Source: CAD feature listing. Evaluate the final solid. Frame: model axes, mm. A direction names the side the tool comes from. Coordinates: 2 decimals unless noted, no trailing zeros. Loops run counter-clockwise (first coordinate to the right, second up) from the corner with the lowest first, then second, coordinate; pieces in that order, holes last. Notation, with made-up numbers: (79, 50) -> (106, 50) arc R24 cw to (106, 71) -> close; hole circle Ø5 at (-10.75, 39). An arc over 180 degrees is marked (long way). Answer as CSV lines item,"result".
from build123d import *

# Parameters (mm, degrees)
BOSS_EXTRUDE1_DEPTH = 20
BOSS_EXTRUDE2_START = 4
BOSS_EXTRUDE2_DEPTH = 4
FILLET1_R           = 4
FILLET2_R           = 3
FILLET3_R           = 2


with BuildPart() as part:
    # Sketch2 → Boss-Extrude1 (new body)
    with BuildSketch(Plane(origin=(0, 0, 0), x_dir=(1, 0, 0), z_dir=(0, 1, 0))):
        with BuildLine():
            Line((9.470598027, 121.732262156), (45.948280407, 88.226297118))
            ThreePointArc((45.948280407, 88.226297118), (47.350268632, 87.077889107), (48.873132869, 86.09539409))
            ThreePointArc((48.873132869, 86.09539409), (0, -99), (-48.873132869, 86.09539409))
            ThreePointArc((-48.873132869, 86.09539409), (-47.350268632, 87.077889107), (-45.948280407, 88.226297118))
            Line((-45.948280407, 88.226297118), (-9.470598027, 121.732262156))
            ThreePointArc((-9.470598027, 121.732262156), (0, 125.42169607), (9.470598027, 121.732262156))
        make_face()
        with BuildLine():
            Line((-6.764712877, 118.786386131), (-43.242395256, 85.280421094))
            ThreePointArc((-43.242395256, 85.280421094), (-44.994880537, 83.84491108), (-46.898460834, 82.616792309))
            ThreePointArc((-46.898460834, 82.616792309), (0, -95), (46.898460834, 82.616792309))
            ThreePointArc((46.898460834, 82.616792309), (44.994880537, 83.84491108), (43.242395256, 85.280421094))
            Line((43.242395256, 85.280421094), (6.764712877, 118.786386131))
            ThreePointArc((6.764712877, 118.786386131), (0, 121.42169607), (-6.764712877, 118.786386131))
        make_face(mode=Mode.SUBTRACT)
    extrude(amount=-BOSS_EXTRUDE1_DEPTH)

    # Sketch2<2> → Boss-Extrude2 (add)
    with BuildSketch(Plane(origin=(0, 0, 0), x_dir=(1, 0, 0), z_dir=(0, 1, 0)).offset(BOSS_EXTRUDE2_START)):
        with BuildLine():
            Line((9.470598027, 121.732262156), (45.948280407, 88.226297118))
            ThreePointArc((45.948280407, 88.226297118), (47.350268632, 87.077889107), (48.873132869, 86.09539409))
            ThreePointArc((48.873132869, 86.09539409), (0, -99), (-48.873132869, 86.09539409))
            ThreePointArc((-48.873132869, 86.09539409), (-47.350268632, 87.077889107), (-45.948280407, 88.226297118))
            Line((-45.948280407, 88.226297118), (-9.470598027, 121.732262156))
            ThreePointArc((-9.470598027, 121.732262156), (0, 125.42169607), (9.470598027, 121.732262156))
        make_face()
    extrude(amount=-BOSS_EXTRUDE2_DEPTH)

    # Fillet1
    fillet1_edges = [part.edges().sort_by_distance(p)[0] for p in [
        (44.994880537, 0, -83.84491108),
        (25.003554066, 0, -102.033403612),
        (0, 0, -121.42169607),
        (-25.003554066, 0, -102.033403612),
        (-44.994880537, 0, -83.84491108),
        (0, 0, 95),
    ]]
    fillet(fillet1_edges, radius=FILLET1_R)

    # Fillet2
    fillet2_edges = [part.edges().sort_by_distance(p)[0] for p in [
        (-47.350268632, 4, -87.077889107),
        (27.709439217, 4, -104.979279637),
        (0, 4, -125.42169607),
        (0, 4, 99),
        (47.350268632, 4, -87.077889107),
        (-27.709439217, 4, -104.979279637),
    ]]
    fillet(fillet2_edges, radius=FILLET2_R)

    # Fillet3
    fillet3_edges = [part.edges().sort_by_distance(p)[0] for p in [
        (47.350268632, -20, -87.077889107),
        (27.709439217, -20, -104.979279637),
        (0, -20, -125.42169607),
        (44.994880537, -20, -83.84491108),
        (0, -20, 95),
        (-44.994880537, -20, -83.84491108),
        (-25.003554066, -20, -102.033403612),
        (0, -20, -121.42169607),
        (25.003554066, -20, -102.033403612),
        (-27.709439217, -20, -104.979279637),
        (-47.350268632, -20, -87.077889107),
        (0, -20, 99),
    ]]
    fillet(fillet3_edges, radius=FILLET3_R - 0.0001)  # a hair under: the kernel refuses the full size


solid = part.part
(1) Pin query (flat end, axial travel): pin 1 Ø3 at (x, z) = (8, -17) entering from -Y; pin 2 Ø6 at (y, z) = (-5.5, -78.5) entering from -X; pin 3 Ø5 at (x, y) = (33.5, -1) entering from -Z. Return the tip coordinate at first contact, or that it passes through.
Computed values:
pin 1,"y = 0"
pin 2,"x = -64.04"
pin 3,"z = -101.96"
(2) Access query for faces 4 (the cylindrical face through (27.6, -19.4, -104.3)), 5 (the cylindrical face through (25.16, -19.43, -102.71)). Directions: +Z, -Z, +X, -X, +Y, -Y. A direction counts if a zero-diameter tool reaches every point of the face in a straight line with its end or side. Return the directions, or none.
Computed values:
face 4,"-Z, +X, -Y"
face 5,"-Y"
(3) Draft query along X for faces 1 (the cylindrical face through (3.638, -8.367, 98.933)), 2 (the cylindrical face through (27.4, 3.1, -104.1)), 3 (the cylindrical face through (23.935, -1.141, -101.382)). Return one class per face: released by +X, released by -X, zero draft, split by the parting line, or undercut.
Computed values:
face 1,"split by the parting line"
face 2,"released by +X"
face 3,"undercut"
(4) Cut plane A-A (y = -7.5). Return the cut outline in (x, z), then the cut area to 3 significant figures.
Computed values:
outline,"(-48.87, -86.1) arc R16 cw to (-45.95, -88.23) -> (-9.47, -121.73) arc R14 ccw to (9.47, -121.73) -> (45.95, -88.23) arc R16 cw to (48.87, -86.1) arc R99 ccw (long way) to start; hole (-46.9, -82.62) arc R20 cw to (-43.24, -85.28) -> (-6.76, -118.79) arc R10 ccw to (6.76, -118.79) -> (43.24, -85.28) arc R20 cw to (46.9, -82.62) arc R95 ccw (long way) to start"
area,"2,540 mm^2"
(5) Material intervals for L1, parallel to X at y = -11.5, z = 0; L2, parallel to Y at x = 73, z = -42.5; L3, parallel to Z at x = -49.5, y = -6.25, sorted ascending. Write a range as [from, to].
Computed values:
L1,"[-99, -95], [95, 99]"
L2,"[0, 4]"
L3,"[-85.74, -81.08], [81.08, 85.74]"
